```python
from build123d import *

# Parameters (mm, degrees)
BOSS_EXTRUDE1_DEPTH = 35.585942761
SKETCH2_R           = 1
BOSS_EXTRUDE2_DEPTH = 8.970038879
BOSS_EXTRUDE3_START = 6.494237864
SKETCH3_R           = 1
BOSS_EXTRUDE3_DEPTH = 6.494237864


with BuildPart() as part:
    # Sketch1 → Boss-Extrude1 (new body)
    with BuildSketch(Plane.XY):
        with BuildLine():
            Line((0, 3.560392335), (0, 4.291474396))
            ThreePointArc((0, 4.291474396), (0.77248629, 4.221376248), (1.519736563, 4.013371808))
            Line((1.519736563, 4.013371808), (1.260839029, 3.329666428))
            ThreePointArc((1.260839029, 3.329666428), (1.932350917, 2.990386849), (2.517577564, 2.517577564))
            Line((2.517577564, 2.517577564), (3.034530647, 3.034530647))
            ThreePointArc((3.034530647, 3.034530647), (3.531194065, 2.438733477), (3.912498451, 1.763266392))
            Line((3.912498451, 1.763266392), (3.245977537, 1.462881883))
            ThreePointArc((3.245977537, 1.462881883), (3.480901257, 0.748144382), (3.560392335, 0))
            Line((3.560392335, 0), (4.291474396, 0))
            ThreePointArc((4.291474396, 0), (4.221376248, -0.77248629), (4.013371808, -1.519736563))
            Line((4.013371808, -1.519736563), (3.329666428, -1.260839029))
            ThreePointArc((3.329666428, -1.260839029), (2.990386849, -1.932350917), (2.517577564, -2.517577564))
            Line((2.517577564, -2.517577564), (3.034530647, -3.034530647))
            ThreePointArc((3.034530647, -3.034530647), (2.438733477, -3.531194065), (1.763266392, -3.912498451))
            Line((1.763266392, -3.912498451), (1.462881883, -3.245977537))
            ThreePointArc((1.462881883, -3.245977537), (0.748144382, -3.480901257), (0, -3.560392335))
            Line((0, -3.560392335), (0, -4.291474396))
            ThreePointArc((0, -4.291474396), (-0.77248629, -4.221376248), (-1.519736563, -4.013371808))
            Line((-1.519736563, -4.013371808), (-1.260839029, -3.329666428))
            ThreePointArc((-1.260839029, -3.329666428), (-1.932350917, -2.990386849), (-2.517577564, -2.517577564))
            Line((-2.517577564, -2.517577564), (-3.034530647, -3.034530647))
            ThreePointArc((-3.034530647, -3.034530647), (-3.531194065, -2.438733477), (-3.912498451, -1.763266392))
            Line((-3.912498451, -1.763266392), (-3.245977537, -1.462881883))
            ThreePointArc((-3.245977537, -1.462881883), (-3.480901257, -0.748144382), (-3.560392335, 0))
            Line((-3.560392335, 0), (-4.291474396, 0))
            ThreePointArc((-4.291474396, 0), (-4.221376248, 0.77248629), (-4.013371808, 1.519736563))
            Line((-4.013371808, 1.519736563), (-3.329666428, 1.260839029))
            ThreePointArc((-3.329666428, 1.260839029), (-2.990386849, 1.932350917), (-2.517577564, 2.517577564))
            Line((-2.517577564, 2.517577564), (-3.034530647, 3.034530647))
            ThreePointArc((-3.034530647, 3.034530647), (-2.438733477, 3.531194065), (-1.763266392, 3.912498451))
            Line((-1.763266392, 3.912498451), (-1.462881883, 3.245977537))
            ThreePointArc((-1.462881883, 3.245977537), (-0.748144382, 3.480901257), (0, 3.560392335))
        make_face()
    extrude(amount=BOSS_EXTRUDE1_DEPTH)

    # Sketch2 → Boss-Extrude2 (add)
    with BuildSketch(Plane.XY.offset(35.585942761)):
        Circle(SKETCH2_R)
    extrude(amount=BOSS_EXTRUDE2_DEPTH)

    # Sketch3 → Boss-Extrude3 (add)
    with BuildSketch(Plane(origin=(0, 0, 0), x_dir=(-1, 0, 0), z_dir=(0, 0, -1)).offset(BOSS_EXTRUDE3_START)):
        with Locations(Location((0, 0, 0), (0, 0, 180))):
            Circle(SKETCH3_R)
    extrude(amount=-BOSS_EXTRUDE3_DEPTH)


solid = part.part
```
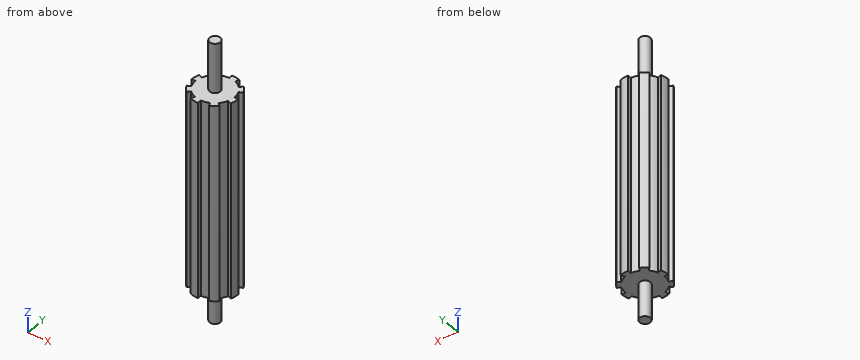
Input: part model. Units: mm. Frame: model coordinates. Round coordinates to 2 decimals unless told otherwise and drop trailing zeros. Loops run counter-clockwise (first coordinate to the right, second up) from the corner with the lowest first, then second, coordinate; pieces in that order, holes last. Notation, with made-up numbers: (88, 26.25) - (147, 26.25) arc R12 cw to (147, 42.25) - close; hole circle Ø2 at (62, 19). An arc over 180 degrees is marked (long way). One line per item, written item: value. Start each with the question number.
(1) Section C-C, the plane z = 40. Return loops of the section in (x, y).
(2) Section B-B, the plane y = 0.5. Return loops of the section in (x, z).
(3) Ray query, line 1 (Z direction, x = -2.75, y = 0.5); line 2 (X direction, y = -0.25, z = 21.5); line 3 (Y direction, x = 3.75, z = 9.5). Return the intervals inside material, ascending. Write a range as [from, to].
(4) Contact query for flat-ended pins moving along their axis: P1, Ø0.8, axis at x = 4, z = 11.5, coming from the +Y side; P2, Ø3, axis at x = 1, y = 3, coming from the +Z side; P3, Ø1, axis at y = -3, z = 19, coming from the -X side. Output: stop coordinate, or through.
Results below:
1. outline: circle Ø2 at (0, 0)
2. outline: (-4.26, 0) - (-0.87, 0) - (-0.87, -6.49) - (0.87, -6.49) - (0.87, 0) - (3.53, 0) - (3.53, 35.59) - (0.87, 35.59) - (0.87, 44.56) - (-0.87, 44.56) - (-0.87, 35.59) - (-4.26, 35.59) - close
3. line 1: [0, 35.59]
3. line 2: [-3.55, 4.28]
3. line 3: [-1.42, 0], [1.69, 2.09]
4. P1: y = 2.34
4. P2: z = 35.59
4. P3: x = -3.49
